Check sheet for the modelled part. Datum: model origin and axes. Units: mm. Face numbers are marked on the shaded views. A direction names the side the tool comes from. Round coordinates to 2 decimals unless told otherwise and drop trailing zeros. Order: outer loops, then holes, each group sorted by start corner. A loop starts at its lowest first (then second) coordinate and runs counter-clockwise, first axis right, second up.
Q1. Cross-section at B-B on x = -1288. Record the cut outline in (y, z), then the cut area to 3 significant figures.
Q2. Set-up check for the marked faces 1 and 2: record each of +Z, -Z, +X, -X, +Y, -Y from which the full face is reachable in a straight line by a thin tool's end or side.
Q3. Scan lines: probe 1 along X at (y, z) = (-295, 77.5); probe 2 along Z at (x, y) = (-1438.5, -846.5); probe 3 along Z at (x, y) = (-237.5, -523). Record each from-to range of solid material in increasing order.
Q4. Cross-section at C-C on z = 706. Record the cut outline in (x, y), then the cut area to 3 significant figures.
Q5. Cross-section at A-A on y = -743.5. Record the cut outline in (x, z), then the cut area to 3 significant figures.
Q6. Depth check by flat-ended pin: P1, Ø1, axis at x = -79.5, y = -483, coming from the -Z side; P2, Ø6, axis at x = -1304, y = -630, coming from the -Z side; P3, Ø2, axis at y = -815.5, z = 265, coming from the -X side. Enter the tip coordinate at first touch or a pass-through.
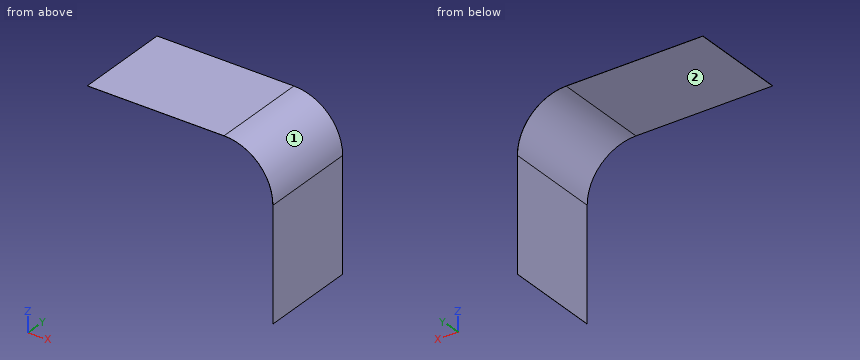
from build123d import *

# Parameters (mm, degrees)
F1_DEPTH = 997.5


with BuildPart() as f1:
    # F0 (on Front) → F1 (new body)
    with BuildSketch(Plane.XZ):
        Polygon((-1648.75, 1648.75), (-950, 1648.75), (-950, 1650), (-1650, 1650), align=None)
        with BuildLine():
            Line((248.75, 1150), (248.75, 0))
            Line((248.75, 0), (250, 0))
            Line((250, 0), (250, 1150))
            ThreePointArc((250, 1150), (103.553391, 1503.553391), (-250, 1650))
            Line((-250, 1650), (-950, 1650))
            Line((-950, 1650), (-950, 1648.75))
            Line((-950, 1648.75), (-250, 1648.75))
            ThreePointArc((-250, 1648.75), (102.669507, 1502.669507), (248.75, 1150))
        make_face()
    extrude(amount=F1_DEPTH)


solid = f1.part
Results found:
1. outline: (-997.5, 1648.75) - (0, 1648.75) - (0, 1650) - (-997.5, 1650) - close
1. area: 1,250 mm2
2. face 1: +Z, +X, +Y, -Y
2. face 2: -Z, -X, +Y, -Y
3. probe 1: x = 248.75 to 250
3. probe 2: z = 1648.75 to 1650
3. probe 3: z = 1648.59 to 1649.84
4. outline: (248.75, -997.5) - (250, -997.5) - (250, 0) - (248.75, 0) - close
4. area: 1,250 mm2
5. outline: (-1650, 1650) - (-1648.75, 1648.75) - (-250, 1648.75) arc R498.75 cw to (248.75, 1150) - (248.75, 0) - (250, 0) - (250, 1150) arc R500 ccw to (-250, 1650) - close
5. area: 4,170 mm2
6. P1: stops at z = 1618.52
6. P2: stops at z = 1648.75
6. P3: stops at x = 248.75
